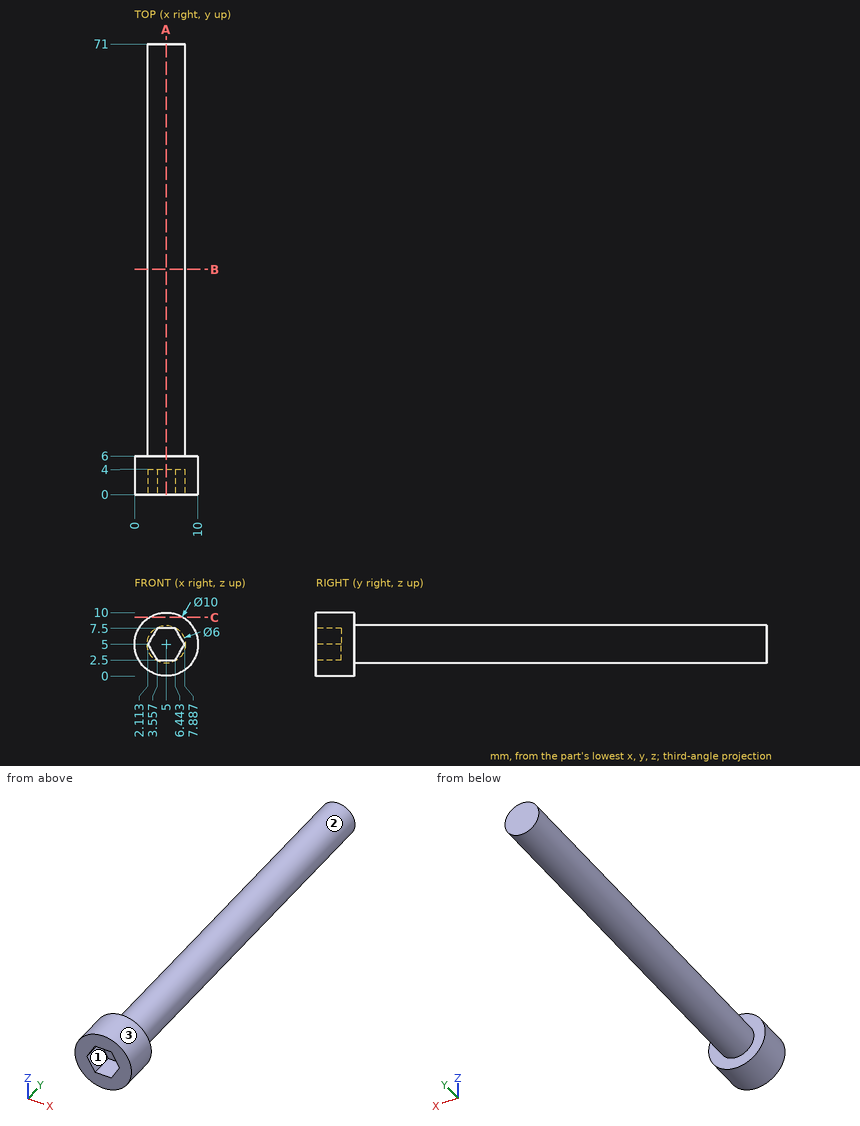
Source: three-view drawing plus pictorial views. Frame: mm from the lowest corner of the part. A direction names the side the tool comes from. Round coordinates to 2 decimals unless told otherwise and drop trailing zeros. Loops run counter-clockwise (first coordinate to the right, second up) from the corner with the lowest first, then second, coordinate; pieces in that order, holes last.
1. Contact query for flat-ended pins moving along their axis: pin 1 (6 mm diameter, centred on x = 7.5, z = 4.5, fed in from -Y); pin 2 (1 mm diameter, centred on x = 4.5, y = 52, fed in from -Z); pin 3 (1.5 mm diameter, centred on y = 59.5, z = 5.5, fed in from -X). Output: stop coordinate, or through.
2. Section query B-B on y = 35.5. Output: boundary loops of the cut face in (x, z).
3. Access query for the marked faces 1, 2 and 3. Directions: +Z, -Z, +X, -X, +Y, -Y. A direction counts if a zero-diameter tool reaches every point of the face in a straight line with its end or side. Return the directions, or none.
4. Section query A-A on x = 5. Output: boundary loops of the cut face in (y, z), and give its area (3 significant figures).
5. Ray query, L1, parallel to Y at x = 3.5, z = 6; L2, parallel to Z at x = 4.75, y = 56.5; L3, parallel to X at y = 9, z = 5. Return the intervals inside material, ascending.
6. Section query C-C on z = 9.25. Output: boundary loops of the cut face in (x, y), and give its area (3 significant figures).
Answers below:
1. pin 1: stops at y = 0
1. pin 2: stops at z = 2
1. pin 3: stops at x = 2
2. outline: circle Ø6 at (5, 5)
3. face 1: -Y
3. face 2: +Y
3. face 3: +Y, -Y
4. outline: (0, 0) - (6, 0) - (6, 2) - (71, 2) - (71, 8) - (6, 8) - (6, 10) - (0, 10) - (0, 7.5) - (4, 7.5) - (4, 2.5) - (0, 2.5) - close
4. area: 430 mm2
5. L1: y = 4 to 71
5. L2: z = 2.01 to 7.99
5. L3: x = 2 to 8
6. outline: (2.37, 0) - (7.63, 0) - (7.63, 6) - (2.37, 6) - close
6. area: 31.6 mm2
